Autodesk Inventor part; units mm, degrees
ref_plane "YZ Plane" through (0, 0, 0) normal (1, 0, 0) x (0, 1, 0)
ref_plane "XZ Plane" through (0, 0, 0) normal (0, 1, 0) x (-1, 0, 0)
ref_plane "XY Plane" through (0, 0, 0) normal (0, 0, 1) x (1, 0, 0)
sketch "Sketch_1" plane through (0, 0, 0) normal (0, 1, 0) x (-1, 0, 0)
  line L0 (-15, 0) -> (0, 0)
  line L1 (0, 0) -> (0, -2.5)
  line L2 (0, -2.5) -> (-0.5, -3)
  line L3 (-0.5, -3) -> (-14.5, -3)
  line L4 (-14.5, -3) -> (-15, -2.5)
  line L5 (-15, -2.5) -> (-15, 0)
  line L6 (-15, 0) -> (0, 0)
revolve "Revolution1" add sketch "Sketch_1" angle 360 about axis through (15, 0, 0) along (1, 0, 0)
sketch "_____9" plane through (0, 0, 3) normal (0, 0, 1) x (1, 0, 0)
  line L0 (0, 1) -> (0, -1)
  line L1 (0, -1) -> (5, -1)
  arc A0 (5, -1) -> (5, 1) centre (5, 0) ccw
  line L2 (5, 1) -> (0, 1)
extrude "Extrusion1" cut sketch "_____9" against normal blind 1.2
sketch "_____14" plane through (0, 0, 3) normal (0, 0, 1) x (1, 0, 0)
  arc A0 (10, 1) -> (10, -1) centre (10, 0) ccw
  line L0 (10, -1) -> (15, -1)
  line L1 (15, -1) -> (15, 1)
  line L2 (15, 1) -> (10, 1)
extrude "Extrusion2" cut sketch "_____14" against normal blind 1.2
properties part number "SSFHKR6-15-KA0-A6-KB9-B6_s"
Check sheet for the modelled part. Datum: model origin and axes. Units: mm. A direction names the side the tool comes from. Give positions to 0.01 mm unless a question says otherwise; leave off trailing zeros. Loops run counter-clockwise (first coordinate to the right, second up) from the corner with the lowest first, then second, coordinate; pieces in that order, holes last. Notation, with made-up numbers: (42, 51.25) - (79, 51.25) arc R29 ccw to (79, 88.25) - close; hole circle Ø10 at (68, 63.5). An arc over 180 degrees is marked (long way). One line per question, with ' | ' between items. Start each with the question number.
1. Set-up check for faces 4 (the flat face through (2, -1, 2)), 5 (the flat face through (13, 1, 2)), 6 (the flat face through (0, 0, 0)): record each of +Z, -Z, +X, -X, +Y, -Y from which the full face is reachable in a straight line by a thin tool's end or side.
2. Gauge pin test, flat ends, axial feed: pin 1 Ø0.5 at (x, z) = (1.5, 2) entering from -Y; pin 2 Ø1.5 at (x, z) = (6, 2) entering from -Y; pin 3 Ø0.6 at (x, y) = (12, -0.5) entering from +Z. Record the tip position at first contact, or that the pin passes through.
3. Cross-section at A-A, the plane y = 0. Enter the section's corners in (x, z), plus the area to 4 significant figures.
4. Draft check along Y on faces 1 (the flat face through (12, -1, 2)), 2 (the conical face through (0.14, -0.1, -2.64)), 3 (the flat face through (15, 0, 0)). Enter one of: released by +Y, released by -Y, zero draft, split by the parting line, or undercut.
5. Material ranges on line 1 along Z through (x, y) = (14.25, 0); line 2 along Y through (x, z) = (10.75, 2.5); line 3 along Y through (x, z) = (13.75, 2.75), recorded low to high. Write a range as [from, to].
6. Cross-section at B-B, the plane x = 11.25. Enter the section's corners in (y, z).
Check result:
1) face 4: +Z, -X | face 5: +Z, +X | face 6: +Z, -Z, -X, +Y, -Y
2) pin 1: stops at y = -2.44 | pin 2: stops at y = -2.73 | pin 3: stops at z = 1.8
3) outline: (0, -2.5) - (0.5, -3) - (14.5, -3) - (15, -2.5) - (15, 1.8) - (9, 1.8) - (9, 3) - (6, 3) - (6, 1.8) - (0, 1.8) - close | area: 75.35 mm2
4) face 1: undercut | face 2: split by the parting line | face 3: zero draft
5) line 1: z = [-3, 1.8] | line 2: y = [-1.66, -1], [1, 1.66] | line 3: y = [-1.2, -1], [1, 1.2]
6) outline: (-1, 1.8) - (-1, 2.83) arc R3 ccw (long way) to (1, 2.83) - (1, 1.8) - close
